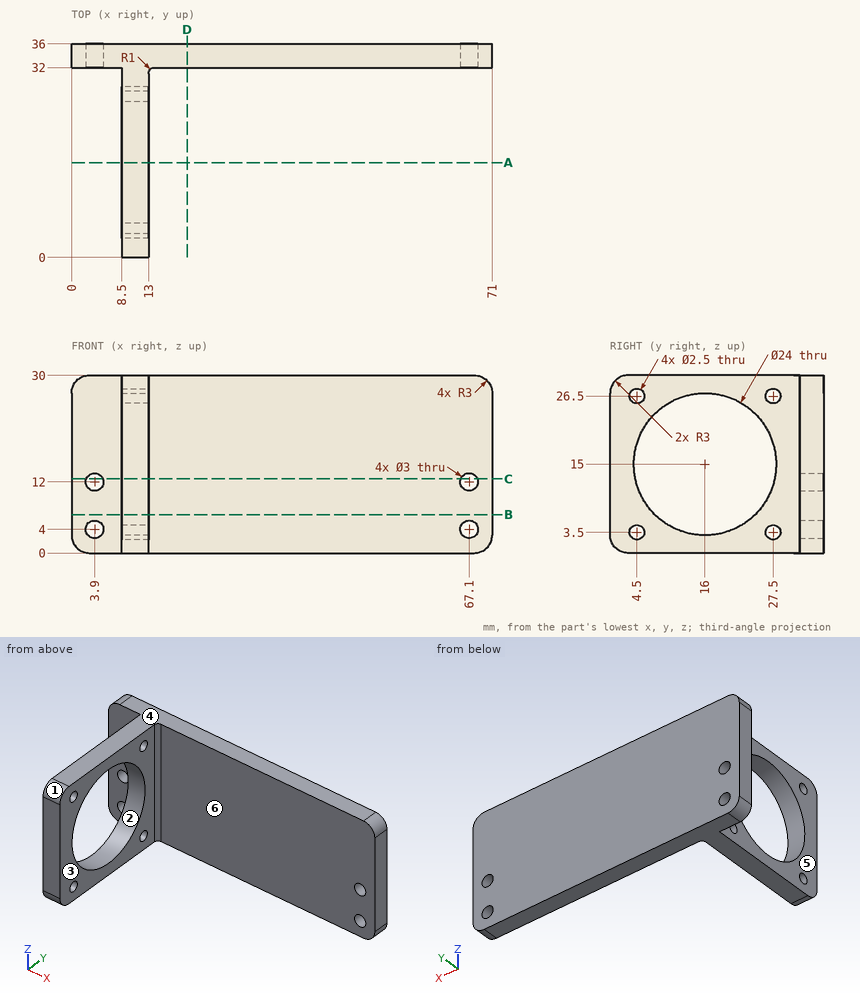
The figure shows three views and two pictorial views of one solid part (mm, origin at its lowest corner). Answer the questions. A direction names the side the tool comes from. Coordinates: 2 decimals unless noted, no trailing zeros. Loops run counter-clockwise (first coordinate to the right, second up) from the corner with the lowest first, then second, coordinate; pieces in that order, holes last. Notation, with made-up numbers: (89.5, 77) - (108.5, 77) arc R20 cw to (108.5, 109) - close; hole circle Ø2 at (-19.5, 57). An arc over 180 degrees is marked (long way). Use a Markdown table: item, result. Add a question column.
1) The part is cut by section D-D, the plane x = 19.5. Give the vertices of the cut face in (y, z), and give its area (3 significant figures).
2) The part is cut by section C-C, the plane z = 12.5. Give the vertices of the cut face in (x, y), and give its area (3 significant figures).
3) The mould has two halves that part along Z. Classify the marked faces 1, 2 and 3: released by +Z, released by -Z, zero draft, split by the parting line, or undercut.
4) Given pin 1 (2 mm diameter, centred on y = 4.5, z = 26.5, fed in from +X); pin 2 (2.5 mm diameter, centred on x = 4, z = 15.5, fed in from -Y); pin 3 (4 mm diameter, centred on y = 27.5, z = 26.5, fed in from +X); pin 4 (12 mm diameter, centred on y = 22.5, z = 15.5, fed in from -X), each flat-ended and moving along its own axis, determine where each tip first touches the part or whether it passes through.
5) The part is cut by section B-B, the plane z = 6.5. Give the vertices of the cut face in (x, y).
6) The part is cut by section A-A, the plane y = 16. Give the vertices of the cut face in (x, z).
7) For the marked faces 4, 5 and 6, determine the directions among +Z, -Z, +X, -X, +Y, -Y from which every point of the face is accessible in a straight line to the end or side of a thin tool.
8) Find the intervals of material crossed by line 1 (Z direction, x = 67, y = 34); line 2 (X direction, y = 33.6, z = 4); line 3 (Y direction, x = 10.65, z = 15), in increasing order.
Here are the results:
| question | item | result |
|---|---|---|
| 1 | outline | (32, 0) - (36, 0) - (36, 30) - (32, 30) - close |
| 1 | area | 120 mm^2 |
| 2 | outline | (0, 32) - (2.49, 32) - (2.49, 36) - (0, 36) - close; (5.31, 32) - (8.5, 32) - (8.5, 27.74) - (13, 27.74) - (13, 31) arc R1 cw to (14, 32) - (65.69, 32) - (65.69, 36) - (5.31, 36) - close; (8.5, 0) - (13, 0) - (13, 4.26) - (8.5, 4.26) - close; (68.51, 32) - (71, 32) - (71, 36) - (68.51, 36) - close |
| 2 | area | 300 mm^2 |
| 3 | face 1 | released by +Z |
| 3 | face 2 | undercut |
| 3 | face 3 | zero draft |
| 4 | pin 1 | passes through |
| 4 | pin 2 | stops at y = 32 |
| 4 | pin 3 | stops at x = 13 |
| 4 | pin 4 | stops at x = 8.5 |
| 5 | outline | (0, 32) - (8.5, 32) - (8.5, 24.47) - (13, 24.47) - (13, 31) arc R1 cw to (14, 32) - (71, 32) - (71, 36) - (0, 36) - close; (8.5, 0) - (13, 0) - (13, 7.53) - (8.5, 7.53) - close |
| 6 | outline | (8.5, 0) - (13, 0) - (13, 3) - (8.5, 3) - close; (8.5, 27) - (13, 27) - (13, 30) - (8.5, 30) - close |
| 7 | face 4 | +Z, +X, -X, +Y, -Y |
| 7 | face 5 | +Z, -Z, -X, -Y |
| 7 | face 6 | +Z, -Z, +X, -Y |
| 8 | line 1 | z = 0 to 2.5, 5.5 to 10.5, 13.5 to 30 |
| 8 | line 2 | x = 0 to 2.4, 5.4 to 65.6, 68.6 to 71 |
| 8 | line 3 | y = 0 to 4, 28 to 36 |
